```python
from build123d import *

# Parameters (mm, degrees)
SKETCH_1_R          = 4
EXTRUDE_1_DEPTH     = 5
SKETCH_2_R          = 4
SKETCH_2_R_2        = 3
EXTRUDE_2_DEPTH     = 3
SKETCH_3_R          = 1.5
CUT_EXTRUDE_1_DEPTH = 10
SKETCH_4_R          = 2.85
CUT_EXTRUDE_2_DEPTH = 3


with BuildPart() as part:
    # 草图1 → 凸台-拉伸1 (new body)
    with BuildSketch(Plane.XY):
        with BuildLine():
            Line((23.05, 8.65181281), (-13.25, 14.530588193))
            ThreePointArc((-13.25, 14.530588193), (-31.25, -0.166350264), (-13.25, -14.86328872))
            Line((-13.25, -14.86328872), (23.05, -8.984513338))
            ThreePointArc((23.05, -8.984513338), (30.25, -0.166350264), (23.05, 8.65181281))
        make_face()
        with Locations((21.25, -0.166350264)):
            Circle(SKETCH_1_R, mode=Mode.SUBTRACT)
        with Locations((-16.25, -0.166350264)):
            Circle(SKETCH_1_R, mode=Mode.SUBTRACT)
    extrude(amount=EXTRUDE_1_DEPTH)

    # 草图2 → 凸台-拉伸2 (add)
    with BuildSketch(Plane(origin=(0, 0, 0), x_dir=(-1, 0, 0), z_dir=(0, 0, -1))):
        with Locations((-21.25, -0.166350264)):
            Circle(SKETCH_2_R)
        with Locations((-21.25, -0.166350264)):
            Circle(SKETCH_2_R_2, mode=Mode.SUBTRACT)
    extrude(amount=-EXTRUDE_2_DEPTH)

    # 草图3 → 切除-拉伸1 (cut)
    with BuildSketch(Plane.XY.offset(5)):
        with Locations((-16.25, 9.733649736)):
            Circle(SKETCH_3_R)
        with Locations((-6.35, -0.166350264)):
            Circle(SKETCH_3_R)
        with Locations((-26.15, -0.166350264)):
            Circle(SKETCH_3_R)
        with Locations((-16.25, -10.066350264)):
            Circle(SKETCH_3_R)
    extrude(amount=-CUT_EXTRUDE_1_DEPTH, mode=Mode.SUBTRACT)

    # 草图4 → 切除-拉伸2 (cut)
    with BuildSketch(Plane.XY.offset(5)):
        with Locations((-16.25, 9.733649736)):
            Circle(SKETCH_4_R)
        with Locations((-26.15, -0.166350264)):
            Circle(SKETCH_4_R)
        with Locations((-6.35, -0.166350264)):
            Circle(SKETCH_4_R)
        with Locations((-16.25, -10.066350264)):
            Circle(SKETCH_4_R)
    extrude(amount=-CUT_EXTRUDE_2_DEPTH, mode=Mode.SUBTRACT)


solid = part.part
```
Can you work these out from the model? Positions are in its coordinate system, mm. A direction names the side the tool comes from. Round coordinates to 2 decimals unless told otherwise and drop trailing zeros. Order: outer loops, then holes, each group sorted by start corner. A loop starts at its lowest first (then second) coordinate and runs counter-clockwise, first axis right, second up. Notation, with made-up numbers: (5, -40) -> (51, -40) arc R24 cw to (51, -8) -> close; hole circle Ø10 at (6.25, 47). An arc over 180 degrees is marked (long way). Return JSON: item names as keys, results as strings. Group by question number.
1. If we section it at C-C, the plane x = -26.15: Write out the boundary of the cut face in (y, z), then the cut area to 3 significant figures.
2. Which directions (+Z, -Z, +X, -X, +Y, -Y) give clear straight access to the entire face, cutting with the end or side of a thin tool? Please do faces 1 (the face through (0, 0, 0)), 2 (the face through (-15, -11.3, 2)).
3. Will these pins go through, and if not, where does the flat tip stop? pin 1 (1.7 mm diameter, centred on x = -17.5, y = -10.5, fed in from +Z); pin 2 (3 mm diameter, centred on y = -10, z = 4, fed in from +X).
4. If we section it at B-B, the plane z = 1.15: Write out the boundary of the cut face in (x, y).
5. If we section it at A-A, the plane x = -16.25: Write out the boundary of the cut face in (y, z).
6. I need wall thicknesses on line 1 (Y direction, x = -16.25, z = 1.65); line 2 (Y direction, x = -16.25, z = 3.5); line 3 (X direction, y = 1.25, z = 2.65). Which ranges of each line are inside material? Lowest first, please. Write a range as [from, to].
7. If we section it at D-D, the plane z = 3.75: Write out the boundary of the cut face in (x, y), then the cut area to 3 significant figures.
8. We'd pull the mould along X, two halves only. Please class faces 3 (the face through (-31.245, 0.206, 2.465)), 4 (the face through (30.25, -0.34, 2.46)), 5 (the face through (18.076, -2.6, 3.986)): released by +X, released by -X, zero draft, split by the parting line, or undercut.
Output values:
{
 "1": {"outline": "(-11.44, 0) -> (-1.67, 0) -> (-1.67, 2) -> (-3.02, 2) -> (-3.02, 5) -> (-11.44, 5) -> close; (1.33, 0) -> (11.1, 0) -> (11.1, 5) -> (2.68, 5) -> (2.68, 2) -> (1.33, 2) -> close", "area": "89.6 mm²"},
 "2": {"face 1": "-Z, +X, -X, +Y, -Y", "face 2": "+Z"},
 "3": {"pin 1": "z = 2", "pin 2": "x = 24.65"},
 "4": {"outline": "(-13.25, -14.86) -> (23.05, -8.98) arc R9 ccw to (23.05, 8.65) -> (-13.25, 14.53) arc R15 ccw (long way) to start; hole circle Ø3 at (-26.15, -0.17); hole circle Ø8 at (-16.25, -0.17); hole circle Ø3 at (-16.25, -10.07); hole circle Ø3 at (-16.25, 9.73); hole circle Ø3 at (-6.35, -0.17); hole circle Ø6 at (21.25, -0.17)"},
 "5": {"outline": "(-15.17, 0) -> (-11.57, 0) -> (-11.57, 2) -> (-12.92, 2) -> (-12.92, 5) -> (-15.17, 5) -> close; (-8.57, 0) -> (-4.17, 0) -> (-4.17, 5) -> (-7.22, 5) -> (-7.22, 2) -> (-8.57, 2) -> close; (3.83, 0) -> (8.23, 0) -> (8.23, 2) -> (6.88, 2) -> (6.88, 5) -> (3.83, 5) -> close; (11.23, 0) -> (14.83, 0) -> (14.83, 5) -> (12.58, 5) -> (12.58, 2) -> (11.23, 2) -> close"},
 "6": {"line 1": "[-15.17, -11.57], [-8.57, -4.17], [3.83, 8.23], [11.23, 14.83]", "line 2": "[-15.17, -12.92], [-7.22, -4.17], [3.83, 6.88], [12.58, 14.83]", "line 3": "[-31.18, -28.62], [-23.68, -19.99], [-12.51, -8.82], [-3.88, 18.61], [23.89, 30.14]"},
 "7": {"outline": "(-13.25, -14.86) -> (23.05, -8.98) arc R9 ccw to (23.05, 8.65) -> (-13.25, 14.53) arc R15 ccw (long way) to start; hole circle Ø5.7 at (-26.15, -0.17); hole circle Ø8 at (-16.25, -0.17); hole circle Ø5.7 at (-16.25, -10.07); hole circle Ø5.7 at (-16.25, 9.73); hole circle Ø5.7 at (-6.35, -0.17); hole circle Ø8 at (21.25, -0.17)", "area": "1,190 mm²"},
 "8": {"face 3": "split by the parting line", "face 4": "released by +X", "face 5": "undercut"}
}
